from build123d import *

# Parameters (mm, degrees)
SCHIZZO1_W                   = 104
SCHIZZO1_H                   = 104
ESTRUSIONE_ESTRUSIONE1_DEPTH = 4
SCHIZZO2_W                   = 100
SCHIZZO2_H                   = 100
TAGLIO_ESTRUSIONE2_DEPTH     = 3
RACCORDO1_R                  = 1
RACCORDO2_R                  = 2


with BuildPart() as part:
    # Schizzo1 → Estrusione-Estrusione1 (new body)
    with BuildSketch(Plane(origin=(0, 0, 0), x_dir=(1, 0, 0), z_dir=(0, 1, 0))):
        Rectangle(SCHIZZO1_W, SCHIZZO1_H)
    extrude(amount=ESTRUSIONE_ESTRUSIONE1_DEPTH)

    # Schizzo2 → Taglio-Estrusione2 (cut)
    with BuildSketch(Plane(origin=(0, 0, 0), x_dir=(1, 0, 0), z_dir=(0, 1, 0))):
        Rectangle(SCHIZZO2_W, SCHIZZO2_H)
    extrude(amount=TAGLIO_ESTRUSIONE2_DEPTH, mode=Mode.SUBTRACT)

    # Raccordo1
    raccordo1_edges = [part.edges().sort_by_distance(p)[0] for p in [
        (0, 4, -52),
        (-52, 4, 0),
        (0, 4, 52),
    ]]
    fillet(raccordo1_edges, radius=RACCORDO1_R)

    # Raccordo2
    # the kernel refuses this fillet: 2 mm, written as the material it takes off along each edge
    with BuildSketch(Plane(origin=(-50, 4, -50), x_dir=(0, 0, -1), z_dir=(1, 0, 0))) as raccordo2_piece_1:
        with BuildLine():
            CenterArc((1, -1), 1, 0, 90)
            Line((2, -1), (2, 0))
            Line((2, 0), (1, 0))
        make_face()
    revolve(axis=Axis((-50, 4, -50), (0, 1, 0)), revolution_arc=90, mode=Mode.SUBTRACT)
    with BuildSketch(Plane(origin=(-50, 4, 50), x_dir=(-1, 0, 0), z_dir=(0, 0, -1))) as raccordo2_piece_2:
        with BuildLine():
            CenterArc((1, -1), 1, 0, 90)
            Line((2, -1), (2, 0))
            Line((2, 0), (1, 0))
        make_face()
    revolve(axis=Axis((-50, 4, 50), (0, 1, 0)), revolution_arc=90, mode=Mode.SUBTRACT)
    with BuildSketch(Plane(origin=(-52, -5, 52), x_dir=(1, 0, 0), z_dir=(0, 1, 0)), Plane(origin=(-52, -5, -52), x_dir=(0, 0, 1), z_dir=(0, 1, 0))) as raccordo2_piece_3:
        with BuildLine():
            CenterArc((RACCORDO2_R, RACCORDO2_R), RACCORDO2_R, 180, 90)
            Line((0, RACCORDO2_R), (0, 0))
            Line((0, 0), (RACCORDO2_R, 0))
        make_face()
    extrude(amount=9, mode=Mode.SUBTRACT)


solid = part.part
Input: part model. Units: mm. Frame: model coordinates. A direction names the side the tool comes from. Coordinates: 2 decimals unless noted, no trailing zeros. Loops run counter-clockwise (first coordinate to the right, second up) from the corner with the lowest first, then second, coordinate; pieces in that order, holes last.
Q1. Material intervals for line 1 (X direction, y = 2.1, z = -2); line 2 (Z direction, x = -27, y = 3.1), sorted ascending.
Q2. Set-up query: faces 1 (the face through (0, 1, -52)), 2 (the face through (50, 1, 1)). Return all of +Z, -Z, +X, -X, +Y, -Y with unobstructed straight access to the full face (end or side cutting, diameter ignored); none if empty.
Q3. Cut plane A-A (y = 0.95). Output: boundary loops of the cut face in (x, z), then the cut area to 3 significant figures.
Q4. Cut plane B-B (z = -31.5). Output: boundary loops of the cut face in (x, y).
Q5. Draft query along X for faces 3 (the face through (-52, 1, 1)), 4 (the face through (-50, 1, 1)), 5 (the face through (52, 2, 1)). Return one class per face: +X half, -X half, draft (parallel to the pull), parting line (faces both ways), or undercut.
Q6. Cut plane C-C (x = -9). Output: boundary loops of the cut face in (y, z), then the cut area to 3 significant figures.
Q7. Contact query for a flat-ended pin moving along its axis: pin 1 (1 mm diameter, centred on x = 10, z = 12.5, fed in from -Y). Output: stop coordinate, or through.
Working result:
1. line 1: x = -52 to -50, 50 to 52
1. line 2: z = -51.99 to 51.99
2. face 1: -Z, +X, -X, +Y, -Y
2. face 2: -Y
3. outline: (-52, -50) arc R2 ccw to (-50, -52) - (52, -52) - (52, 52) - (-50, 52) arc R2 ccw to (-52, 50) - close; hole (-50, -50) - (50, -50) - (50, 50) - (-50, 50) - close
3. area: 814 mm2
4. outline: (-52, 0) - (-50, 0) - (-50, 3) - (50, 3) - (50, 0) - (52, 0) - (52, 4) - (-51, 4) arc R1 ccw to (-52, 3) - close
5. face 3: -X half
5. face 4: undercut
5. face 5: +X half
6. outline: (0, -52) - (3, -52) arc R1 ccw to (4, -51) - (4, 51) arc R1 ccw to (3, 52) - (0, 52) - (0, 50) - (3, 50) - (3, -50) - (0, -50) - close
6. area: 116 mm2
7. pin 1: stops at y = 3
